```python
from build123d import *

# Parameters (mm, degrees)
F1_DEPTH = 1.6
F2_R     = 3.3061205596
F2_R_2   = 3.3042251001
F3_DEPTH = 8


# Not quite as in the source:
# - ends of sketch curves that miss each other by under 0.0002 mm in the source are joined


with BuildPart() as f1:
    # F0 (on Top) → F1 (new body)
    with BuildSketch(Plane.XY):
        with BuildLine():
            Line((-30.10027, 26.72715), (-30.10027, -23.27275))
            ThreePointArc((-30.10027, -23.27275), (-29.2216664958, -25.3938864958), (-27.10053, -26.27249))
            Line((-27.10053, -26.27249), (-24.63927, -26.27249))
            Line((-24.63927, -26.27249), (-23.36927, -25.00249))
            Line((-23.36927, -25.00249), (-3.30327, -25.00249))
            Line((-3.30327, -25.00249), (-2.03327, -26.27249))
            Line((-2.03327, -26.27249), (31.89859, -26.27249))
            ThreePointArc((31.89859, -26.27249), (34.020096129, -25.3935121782), (34.9008668601, -23.2727499955))
            Line((34.9008668601, -23.2727499955), (34.90087, 26.72715))
            ThreePointArc((34.90087, 26.72715), (34.0213682803, 28.8491843311), (31.8985900009, 29.7268889246))
            Line((31.8985900009, 29.7268889246), (-27.10053, 29.72689))
            ThreePointArc((-27.10053, 29.72689), (-29.2216664958, 28.8482864958), (-30.10027, 26.72715))
        make_face()
        with BuildLine():
            ThreePointArc((-26.60015, -24.14651), (-27.5718137123, -23.7440337123), (-27.97429, -22.77237))
            ThreePointArc((-27.97429, -22.77237), (-27.5718137123, -21.8007062877), (-26.60015, -21.39823))
            ThreePointArc((-26.60015, -21.39823), (-25.6284862877, -21.8007062877), (-25.22601, -22.77237))
            ThreePointArc((-25.22601, -22.77237), (-25.6284862877, -23.7440337123), (-26.60015, -24.14651))
        make_face(mode=Mode.SUBTRACT)
        with BuildLine():
            ThreePointArc((31.40075, -24.14651), (30.4290862877, -23.7440337123), (30.02661, -22.77237))
            ThreePointArc((30.02661, -22.77237), (30.4290862877, -21.8007062877), (31.40075, -21.39823))
            ThreePointArc((31.40075, -21.39823), (32.3724137123, -21.8007062877), (32.77489, -22.77237))
            ThreePointArc((32.77489, -22.77237), (32.3724137123, -23.7440337123), (31.40075, -24.14651))
        make_face(mode=Mode.SUBTRACT)
        with BuildLine():
            ThreePointArc((-26.60015, 24.8538994131), (-27.5713650107, 25.2559269636), (-27.97429, 26.22677))
            ThreePointArc((-27.97429, 26.22677), (-27.5722630364, 27.1992550107), (-26.60015, 27.6021805869))
            ThreePointArc((-26.60015, 27.6021805869), (-25.6284858727, 27.1997041273), (-25.2260094131, 26.22804))
            ThreePointArc((-25.2260094131, 26.22804), (-25.2260095598, 26.2274049999), (-25.22601, 26.22677))
            ThreePointArc((-25.22601, 26.22677), (-25.6289349893, 25.2559269636), (-26.60015, 24.8538994131))
        make_face(mode=Mode.SUBTRACT)
        with BuildLine():
            ThreePointArc((32.77489, 26.22677), (31.39948, 24.85136), (30.02407, 26.22677))
            ThreePointArc((30.02407, 26.22677), (30.4273673786, 27.1997806471), (31.40075, 27.6021794137))
            ThreePointArc((31.40075, 27.6021794137), (32.3724906471, 27.1988826214), (32.77489, 26.22677))
        make_face(mode=Mode.SUBTRACT)
    extrude(amount=F1_DEPTH)

    # F2 (on face) → F3 (join)
    with BuildSketch(Plane.XY.offset(1.6)):
        with Locations((-18.8942644745, -2.7409724426)):
            Circle(F2_R)
        with Locations((-10.6140207499, -2.4052869994)):
            Circle(F2_R_2)
    extrude(amount=F3_DEPTH)


solid = f1.part
```
Here's how the part is built. I have some questions about the finished solid (model axes, mm). A direction names the side the tool comes from. Coordinates: 2 decimals unless noted, no trailing zeros. Order: outer loops, then holes, each group sorted by start corner. A loop starts at its lowest first (then second) coordinate and runs counter-clockwise, first axis right, second up. Notation, with made-up numbers: (84.25, 20.25) -> (99.25, 20.25) arc R22 ccw to (99.25, 58.25) -> close; hole circle Ø4 at (-37, -27.75). An arc over 180 degrees is marked (long way). Return JSON: item names as keys, results as strings.
1) If we section it at A-A on x = -20.5: List the corners of the cut face in (y, z) for me.
Conclusion:
{"outline": "(-25, 0) -> (29.73, 0) -> (29.73, 1.6) -> (0.15, 1.6) -> (0.15, 9.6) -> (-5.63, 9.6) -> (-5.63, 1.6) -> (-25, 1.6) -> close"}
2) If we section it at D-D on x = -5: List the corners of the cut face in (y, z) for me.
Conclusion:
{"outline": "(-25, 0) -> (29.73, 0) -> (29.73, 1.6) -> (-25, 1.6) -> close"}
3) On a 3-axis mill with a long thin cutter (end or side, diameter ignored), from which of +Z, -Z, +X, -X, +Y, -Y can I reach the whole of each face in a straight line? I mean faces 4 (the flat face through (34.901, 1, 1)), 5 (the cylindrical face through (-15.74, -1.75, 5.54)), 6 (the flat face through (-13, -25.002, 1)). Say none if no direction works.
Conclusion:
{"face 4": "+Z, -Z, +X, +Y, -Y", "face 5": "+Z", "face 6": "+Z, -Z, -Y"}
4) If we section it at C-C on z = 2.75: List the corners of the cut face in (x, y) for me.
Conclusion:
{"outline": "circle Ø6.61 at (-18.89, -2.74); circle Ø6.61 at (-10.61, -2.41)"}
5) Thinking about a two-plate mould opening in X: for faces 1 (the cylindrical face through (-29.245, -25.37, 0.789)), 2 (the cylindrical face through (-13.236, -4.416, 5.544)), 3 (the cylindrical face through (33.997, -25.417, 0.789)), which applies, +X half, -X half, draft (parallel to the pull), parting line (faces both ways), or undercut?
Conclusion:
{"face 1": "-X half", "face 2": "undercut", "face 3": "+X half"}
6) If we section it at B-B on y = 18: List the corners of the cut face in (x, z) for me, plus the area to 3 significant figures.
Conclusion:
{"outline": "(-30.1, 0) -> (34.9, 0) -> (34.9, 1.6) -> (-30.1, 1.6) -> close", "area": "104 mm²"}
7) I'm going to push flat-ended pins straight in: P1, Ø12, axis at x = -8, y = -14, coming from the +Z side; P2, Ø1, axis at y = 22.5, z = 2.5, coming from the +X side; P3, Ø0.8, axis at x = -13.5, z = 1, coming from the -Y side. Where does each tip first touch, or does it pass through?
Conclusion:
{"P1": "stops at z = 1.6", "P2": "passes through", "P3": "stops at y = -25"}
8) If I drill on probe 1 along X at (y, z) = (-24, 1); probe 2 along Z at (x, y) = (2, -6); probe 3 along Y at (x, z) = (-21, 1), over which ranges is the centre line in solid material (lowest first)?
Conclusion:
{"probe 1": "x = -30.01 to -27.22, -25.98 to 30.78, 32.02 to 34.81", "probe 2": "z = 0 to 1.6", "probe 3": "y = -25 to 29.73"}
